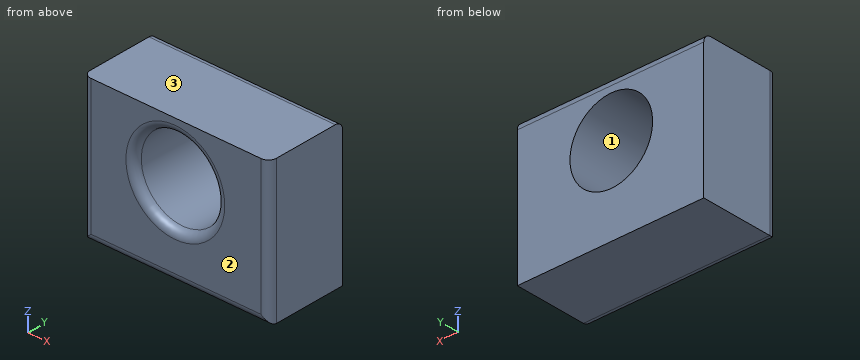
from build123d import *

# Parameters (mm, degrees)
F0_W     = 117.274408
F0_H     = 89.918245
F0_R     = 26.007652
F1_DEPTH = 50.8
F2_R     = 5.08
F3_R     = 5.08
F4_R     = 5.08


with BuildPart() as f1:
    # F0 (on Front) → F1 (new body)
    with BuildSketch(Plane.XZ):
        with Locations((0.464147, -9.922528)):
            Rectangle(F0_W, F0_H)
        Circle(F0_R, mode=Mode.SUBTRACT)
    extrude(amount=F1_DEPTH)

    # F2
    f2_edges = [f1.edges().sort_by_distance(p)[0] for p in [
        (0.464147, 0, 35.036594),
    ]]
    fillet(f2_edges, radius=F2_R)

    # F3
    f3_edges = [f1.edges().sort_by_distance(p)[0] for p in [
        (0.464147, -50.8, -54.881651),
        (-58.173057, -50.8, -9.922529),
        (59.101351, -50.8, -9.922529),
    ]]
    fillet(f3_edges, radius=F3_R)

    # F4
    f4_edges = [f1.edges().sort_by_distance(p)[0] for p in [
        (-26.007652, -50.8, 0),
    ]]
    fillet(f4_edges, radius=F4_R)


solid = f1.part
Here's how the part is built. I have some questions about the finished solid (model axes, mm). Face numbers are marked on the shaded views. Coordinates: 2 decimals unless noted, no trailing zeros. Loops run counter-clockwise (first coordinate to the right, second up) from the corner with the lowest first, then second, coordinate; pieces in that order, holes last.
1. For P1, Ø1.5, axis at x = 24, z = 10, coming from the -Y side, with a flat end and sliding along its axis, tell me the tip position at first contact or that it passes through.
2. I need wall thicknesses on L1, parallel to Z at x = 0, y = -9.5; L2, parallel to X at y = -5.5, z = 4; L3, parallel to Z at x = -15.5, y = -13. Which ranges of each line are inside material? Lowest first, please.
3. Imagine slicing it at B-B, the plane x = 0. Please give me the cut outline in (y, z).
4. If we mould it in two halves opening along Z, with no side actions, what happens to the marked faces 1, 2 and 3? For each: pulls with the +Z half, pulls with the -Z half, needs draft (parallel to the pull), parting line crosses it, or undercut.
5. Imagine slicing it at A-A, the plane z = 0. Please give me the cut outline in (x, y), and give its area (3 significant figures).
6. Imagine slicing it at C-C, the plane y = -32. Please give me the cut outline in (x, z), and give its area (3 significant figures).
Taken from the geometry:
1. P1: stops at y = -48.36
2. L1: z = -54.88 to -26.01, 26.01 to 35.04
2. L2: x = -58.17 to -25.7, 25.7 to 59.1
2. L3: z = -54.88 to -20.88, 20.88 to 35.04
3. outline: (-50.8, -49.8) arc R5.08 ccw to (-45.72, -54.88) - (0, -54.88) - (0, -26.01) - (-45.72, -26.01) arc R5.08 ccw to (-50.8, -31.09) - close; (-50.8, 31.09) arc R5.08 ccw to (-45.72, 26.01) - (0, 26.01) - (0, 29.96) arc R5.08 ccw to (-5.08, 35.04) - (-50.8, 35.04) - close
4. face 1: undercut
4. face 2: needs draft
4. face 3: pulls with the +Z half
5. outline: (-58.17, -45.72) arc R5.08 ccw to (-53.09, -50.8) - (-31.09, -50.8) arc R5.08 ccw to (-26.01, -45.72) - (-26.01, 0) - (-58.17, 0) - close; (26.01, -45.72) arc R5.08 ccw to (31.09, -50.8) - (54.02, -50.8) arc R5.08 ccw to (59.1, -45.72) - (59.1, 0) - (26.01, 0) - close
5. area: 3,290 mm2
6. outline: (-58.17, -54.88) - (59.1, -54.88) - (59.1, 35.04) - (-58.17, 35.04) - close; hole circle Ø52.02 at (0, 0)
6. area: 8,420 mm2
